Autodesk Inventor part; units mm, degrees
ref_plane "YZ Plane" through (0, 0, 0) normal (1, 0, 0) x (0, 1, 0)
ref_plane "XZ Plane" through (0, 0, 0) normal (0, 1, 0) x (-1, 0, 0)
ref_plane "XY Plane" through (0, 0, 0) normal (0, 0, 1) x (1, 0, 0)
sketch "Sketch1" plane through (0, 0, 0) normal (0, 1, 0) x (-1, 0, 0)
  line L0 (0, 0) -> (7, 0)
  line L1 (7, 0) -> (7, -4)
  line L2 (7, -4) -> (0, -4)
  line L3 (0, -4) -> (0, 0)
  line L4 (0, -22.5) -> (26.9418, -22.5) construction
  line L5 (24.5, 0) -> (31.5, 0)
  line L6 (31.5, 0) -> (31.5, -4)
  line L7 (31.5, -4) -> (24.5, -4)
  line L8 (24.5, -4) -> (24.5, 0)
  line L9 (0, -45) -> (7, -45)
  line L10 (7, -45) -> (7, -41)
  line L11 (7, -41) -> (0, -41)
  line L12 (0, -41) -> (0, -45)
  line L13 (24.5, -45) -> (31.5, -45)
  line L14 (31.5, -45) -> (31.5, -41)
  line L15 (31.5, -41) -> (24.5, -41)
  line L16 (24.5, -41) -> (24.5, -45)
  dimension "d0" = 7
  dimension "d1" = 4
  dimension "d2" = 18.5
  dimension "d3" = 7
  dimension "d4" = 17.5
  dimension "d5" = 37
  dimension "d15" = 4
extrude "Extrusion1" add sketch "Sketch1" along normal blind 4.5
sketch "Sketch2" plane through (0, 0, -4) normal (0, 0, -1) x (-1, 0, 0)
  line L0 (0, 0) -> (7, 0)
  line L1 (31.5, 0) -> (31.5, 4.5)
  line L2 (0, 0) -> (31.5, 0)
  line L3 (31.5, 0) -> (31.5, 1.5)
  line L4 (31.5, 1.5) -> (0, 1.5)
  line L5 (0, 1.5) -> (0, 0)
  dimension "d8" = 1.5
  dimension "d11" = 31.5
extrude "Extrusion2" add sketch "Sketch2" along normal blind 37
sketch "Sketch3" plane through (0, 0, 0) normal (0, -1, 0) x (1, 0, 0)
  point P0 (0, 0)
sketch "Sketch4" plane through (-31.5, 0, 0) normal (-1, 0, 0) x (0, 0, 1)
  line L0 (-41, 1.5) -> (-41, 4.5)
  line L1 (0, 0) -> (-45, 0)
  line L2 (-41, 1.5) -> (-4, 1.5)
  line L3 (-4, 1.5) -> (-4, 0)
  line L4 (-4, 0) -> (-41, 0)
  line L5 (-41, 0) -> (-41, 1.5)
  point P0 (-41, 0)
  dimension "d12" = 37
extrude "Extrusion3" add sketch "Sketch4" along normal blind 30
sketch "Sketch5" plane through (-24.5, 1.5, -4) normal (0, 1, 0) x (1, 0, 0)
  circle A0 centre (12.2952, 27.39) radius 0.9
  line L0 (24.5, -4) -> (24.5, 41) construction
  line L1 (24.5, 18.5) -> (-15.4775, 18.5) construction
  circle A1 centre (-33.4248, 27.39) radius 0.9
  circle A2 centre (12.2952, 9.61) radius 0.9
  circle A3 centre (-33.4248, 9.61) radius 0.9
  dimension "d16" = 1.8
  dimension "d17" = 8.89
  dimension "d18" = 1.8
  dimension "d19" = 45.72
  dimension "d22" = 8.89
extrude "Extrusion4" add sketch "Sketch5" along normal blind 3
equation "\"d3\" = d0"
equation "\"d18\" = d16"
equation "\"d22\" = d17"
properties part number "b"
Here's how the part is built. I have some questions about the finished solid (model axes, mm). A direction names the side the tool comes from. Coordinates: 2 decimals unless noted, no trailing zeros. Loops run counter-clockwise (first coordinate to the right, second up) from the corner with the lowest first, then second, coordinate; pieces in that order, holes last. Notation, with made-up numbers: (44, 59) -> (83, 59) arc R16 ccw to (83, 75) -> close; hole circle Ø1 at (32.5, 37). An arc over 180 degrees is marked (long way). Use one line per item in the form item = value. Start each with the question number.
(1) Will these pins go through, and if not, where does the flat tip stop? pin 1 (6 mm diameter, centred on x = -15, z = -31, fed in from +Y); pin 2 (1.2 mm diameter, centred on x = -46.5, y = 1, fed in from -Z); pin 3 (1.6 mm diameter, centred on x = -45.5, y = 0.5, fed in from +Z); pin 4 (2 mm diameter, centred on y = 2.5, z = -44, fed in from -X).
(2) If we section it at A-A (y = 3.75): Please give me the cut outline in (x, z), then the cut area to 3 significant figures.
(3) If we section it at B-B (z = -13.61): Please give me the cut outline in (x, y), then the cut area to 3 significant figures.
(4) If we section it at D-D (x = -50): Please give me the cut outline in (y, z).
(5) Please list where these lines run through material, in increasing order: line 1 along X through (y, z) = (0.3, -3); line 2 along Y through (x, z) = (-50, -24.5); line 3 along X through (y, z) = (2.1, -14).
(6) On a 3-axis mill with a long thin cutter (end or side, diameter ignored), from which of +Z, -Z, +X, -X, +Y, -Y can I reach the whole of each face in a straight line? I mean faces 4 (the face through (-31.5, 2, -43)), 5 (the face through (-7, 2, -43)), 6 (the face through (-16, 1, -4)), 7 (the face through (-57.51, 2.98, -32.19)), 8 (the face through (-28, 3, -4)). Say none if no direction works.
(7) We'd pull the mould along Z, two halves only. Please class faces 1 (the face through (-28, 2, 0)), 2 (the face through (-28, 3, -41)), 3 (the face through (-28, 4.5, -2)): pulls with the +Z half, pulls with the -Z half, needs draft (parallel to the pull), parting line crosses it, or undercut.
(8) If we section it at C-C (y = 0.8): Please give me the cut outline in (x, z), then the cut area to 3 significant figures.
Verdict:
q1.pin_1 = 4.5
q1.pin_2 = -41
q1.pin_3 = -4
q1.pin_4 = -31.5
q2.outline = circle Ø1.8 at (-57.92, -31.39); circle Ø1.8 at (-57.92, -13.61); (-31.5, -45) -> (-24.5, -45) -> (-24.5, -41) -> (-31.5, -41) -> close; (-31.5, -4) -> (-24.5, -4) -> (-24.5, 0) -> (-31.5, 0) -> close; circle Ø1.8 at (-12.2, -31.39); circle Ø1.8 at (-12.2, -13.61); (-7, -45) -> (0, -45) -> (0, -41) -> (-7, -41) -> close; (-7, -4) -> (0, -4) -> (0, 0) -> (-7, 0) -> close
q2.area = 122 mm²
q3.outline = (-61.5, 0) -> (0, 0) -> (0, 1.5) -> (-11.3, 1.5) -> (-11.3, 4.5) -> (-13.1, 4.5) -> (-13.1, 1.5) -> (-57.02, 1.5) -> (-57.02, 4.5) -> (-58.82, 4.5) -> (-58.82, 1.5) -> (-61.5, 1.5) -> close
q3.area = 103 mm²
q4.outline = (0, -41) -> (1.5, -41) -> (1.5, -4) -> (0, -4) -> close
q5.line_1 = -31.5 to -24.5, -7 to 0
q5.line_2 = 0 to 1.5
q5.line_3 = -58.74 to -57.11, -13.02 to -11.39
q6.face_4 = -Z, -X, +Y, -Y
q6.face_5 = -Z, +Y, -Y
q6.face_6 = +Z, +Y, -Y
q6.face_7 = +Y
q6.face_8 = +X, -X, +Y
q7.face_1 = pulls with the +Z half
q7.face_2 = undercut
q7.face_3 = needs draft
q8.outline = (-61.5, -41) -> (-31.5, -41) -> (-31.5, -45) -> (-24.5, -45) -> (-24.5, -41) -> (-7, -41) -> (-7, -45) -> (0, -45) -> (0, 0) -> (-7, 0) -> (-7, -4) -> (-24.5, -4) -> (-24.5, 0) -> (-31.5, 0) -> (-31.5, -4) -> (-61.5, -4) -> close
q8.area = 2,390 mm²
